Geometry: final body of the model. Coordinates: model frame, mm. A direction names the side the tool comes from. Round coordinates to 2 decimals unless told otherwise and drop trailing zeros. Order: outer loops, then holes, each group sorted by start corner. A loop starts at its lowest first (then second) coordinate and runs counter-clockwise, first axis right, second up. Notation, with made-up numbers: M 19.25,-16.75 L 53.25,-16.75 A10 cw 53.25,-7.75 Z; hole C 29,53 d8. An arc over 180 degrees is marked long. Return JSON: item names as keys, results as strings. Group by question number.
Q1. Mould query, pull axis X, two halves, no side actions, for faces 1 (the face through (42, 0, -136)), 2 (the face through (41, 3, -201.308)), 3 (the face through (87.336, 2, -136)), 4 (the face through (67, 3, -260.308)). Classes: released by +X, released by -X, zero draft, split by the parting line, or undercut.
Q2. Cut plane C-C on z = -68. Output: boundary loops of the cut face in (x, y), and give its area (3 significant figures).
Q3. Cut plane D-D on x = 32. Output: boundary loops of the cut face in (y, z), and give its area (3 significant figures).
Q4. Cut plane A-A on x = 20. Output: boundary loops of the cut face in (y, z), and give its area (3 significant figures).
Q5. Contact query for flat-ended pins moving along their axis: pin 1 (2.5 mm diameter, centred on x = 25.34, z = -194.31, fed in from -Y); pin 2 (5 mm diameter, centred on x = 25.34, z = -174.31, fed in from -Y). Output: stop coordinate, or through.
Q6. Ray query, probe 1 along Z at (x, y) = (46, 4.5); probe 2 along Z at (x, y) = (65, 2.4); probe 3 along X at (y, z) = (1, -227). Return the intervals inside material, ascending.
Q7. Cut plane B-B on z = -27. Output: boundary loops of the cut face in (x, y), and give its area (3 significant figures).
Q8. Access query for faces 5 (the face through (5.336, 3, -216)), 6 (the face through (42, 5, -136)). Directions: +Z, -Z, +X, -X, +Y, -Y. A direction counts if a zero-diameter tool reaches every point of the face in a straight line with its end or side. Return the directions, or none.
Autodesk Inventor part; units mm, degrees
ref_plane "YZ Plane" through (0, 0, 0) normal (1, 0, 0) x (0, 1, 0)
ref_plane "XZ Plane" through (0, 0, 0) normal (0, 1, 0) x (-1, 0, 0)
ref_plane "XY Plane" through (0, 0, 0) normal (0, 0, 1) x (1, 0, 0)
sketch "Sketch1" plane through (0, 0, 0) normal (0, 1, 0) x (-1, 0, 0)
  line L0 (4.6641, 6.6919) -> (-87.3359, 6.6919)
  line L1 (-87.3359, 6.6919) -> (-87.3359, -283.3081)
  line L2 (-87.3359, -283.3081) -> (4.6641, -283.3081)
  line L3 (4.6641, -283.3081) -> (4.6641, 6.6919)
  point P0 (0, 0)
  dimension "d0" = 290
  dimension "d1" = 92
extrude "Extrusion1" add sketch "Sketch1" along normal blind 5
sketch "Sketch2" plane through (0, 5, 0) normal (0, 1, 0) x (1, 0, 0)
  line L0 (-4.6641, 283.3081) -> (-4.6641, -6.6919)
  line L1 (87.3359, -6.6919) -> (87.3359, 283.3081)
  line L2 (9.3359, 45.3081) -> (73.3359, 45.3081)
  line L3 (77.3359, 49.3081) -> (77.3359, 71.3081)
  line L4 (73.3359, 75.3081) -> (9.3359, 75.3081)
  line L5 (5.3359, 71.3081) -> (5.3359, 49.3081)
  line L6 (-4.6641, -6.6919) -> (87.3359, -6.6919)
  arc A0 (5.3359, 49.3081) -> (9.3359, 45.3081) centre (9.3359, 49.3081) ccw
  arc A1 (9.3359, 75.3081) -> (5.3359, 71.3081) centre (9.3359, 71.3081) ccw
  arc A2 (77.3359, 71.3081) -> (73.3359, 75.3081) centre (73.3359, 71.3081) ccw
  arc A3 (73.3359, 45.3081) -> (77.3359, 49.3081) centre (73.3359, 49.3081) ccw
  line L7 (9.3359, 201.3081) -> (73.3359, 201.3081)
  line L8 (77.3359, 205.3081) -> (77.3359, 227.3081)
  line L9 (73.3359, 231.3081) -> (9.3359, 231.3081)
  line L10 (5.3359, 227.3081) -> (5.3359, 205.3081)
  arc A4 (5.3359, 205.3081) -> (9.3359, 201.3081) centre (9.3359, 205.3081) ccw
  arc A5 (9.3359, 231.3081) -> (5.3359, 227.3081) centre (9.3359, 227.3081) ccw
  arc A6 (77.3359, 227.3081) -> (73.3359, 231.3081) centre (73.3359, 227.3081) ccw
  arc A7 (73.3359, 201.3081) -> (77.3359, 205.3081) centre (73.3359, 205.3081) ccw
  line L11 (7.3359, 1.3081) -> (75.3359, 1.3081)
  line L12 (77.3359, 3.3081) -> (77.3359, 14.3081)
  line L13 (75.3359, 16.3081) -> (58.3359, 16.3081)
  line L14 (56.3359, 18.3081) -> (56.3359, 35.3081)
  line L15 (54.3359, 37.3081) -> (28.3359, 37.3081)
  line L16 (26.3359, 35.3081) -> (26.3359, 18.3081)
  line L17 (24.3359, 16.3081) -> (7.3359, 16.3081)
  line L18 (5.3359, 14.3081) -> (5.3359, 3.3081)
  arc A8 (5.3359, 3.3081) -> (7.3359, 1.3081) centre (7.3359, 3.3081) ccw
  arc A9 (7.3359, 16.3081) -> (5.3359, 14.3081) centre (7.3359, 14.3081) ccw
  arc A10 (24.3359, 16.3081) -> (26.3359, 18.3081) centre (24.3359, 18.3081) ccw
  arc A11 (28.3359, 37.3081) -> (26.3359, 35.3081) centre (28.3359, 35.3081) ccw
  arc A12 (56.3359, 35.3081) -> (54.3359, 37.3081) centre (54.3359, 35.3081) ccw
  arc A13 (56.3359, 18.3081) -> (58.3359, 16.3081) centre (58.3359, 18.3081) ccw
  arc A14 (77.3359, 14.3081) -> (75.3359, 16.3081) centre (75.3359, 14.3081) ccw
  arc A15 (75.3359, 1.3081) -> (77.3359, 3.3081) centre (75.3359, 3.3081) ccw
  line L19 (87.3359, 283.3081) -> (-4.6641, 283.3081)
  line L20 (5.3359, 273.3081) -> (5.3359, 262.3081)
  line L21 (7.3359, 260.3081) -> (24.3359, 260.3081)
  line L22 (26.3359, 258.3081) -> (26.3359, 241.3081)
  line L23 (28.3359, 239.3081) -> (54.3359, 239.3081)
  line L24 (56.3359, 241.3081) -> (56.3359, 258.3081)
  line L25 (58.3359, 260.3081) -> (75.3359, 260.3081)
  line L26 (77.3359, 262.3081) -> (77.3359, 273.3081)
  line L27 (75.3359, 275.3081) -> (7.3359, 275.3081)
  arc A16 (26.3359, 258.3081) -> (24.3359, 260.3081) centre (24.3359, 258.3081) ccw
  arc A17 (5.3359, 262.3081) -> (7.3359, 260.3081) centre (7.3359, 262.3081) ccw
  arc A18 (7.3359, 275.3081) -> (5.3359, 273.3081) centre (7.3359, 273.3081) ccw
  arc A19 (77.3359, 273.3081) -> (75.3359, 275.3081) centre (75.3359, 273.3081) ccw
  arc A20 (75.3359, 260.3081) -> (77.3359, 262.3081) centre (75.3359, 262.3081) ccw
  arc A21 (58.3359, 260.3081) -> (56.3359, 258.3081) centre (58.3359, 258.3081) ccw
  arc A22 (54.3359, 239.3081) -> (56.3359, 241.3081) centre (54.3359, 241.3081) ccw
  arc A23 (26.3359, 241.3081) -> (28.3359, 239.3081) centre (28.3359, 241.3081) ccw
  point P0 (5.3359, 45.3081)
  point P1 (77.3359, 75.3081)
  point P2 (5.3359, 75.3081)
  point P3 (5.3359, 201.3081)
  point P4 (77.3359, 201.3081)
  point P5 (5.3359, 231.3081)
  point P6 (5.3359, 1.3081)
  point P7 (77.3359, 1.3081)
  point P8 (77.3359, 16.3081)
  point P9 (56.3359, 16.3081)
  point P10 (26.3359, 16.3081)
  point P11 (5.3359, 16.3081)
  point P12 (5.3359, 275.3081)
  point P13 (5.3359, 260.3081)
  point P14 (26.3359, 260.3081)
  point P15 (56.3359, 260.3081)
  point P16 (77.3359, 260.3081)
  point P17 (77.3359, 275.3081)
  dimension "d12" = 30
  dimension "d13" = 72
  dimension "d14" = 10
  dimension "d16" = 4
  dimension "d17" = 30
  dimension "d18" = 10
  dimension "d19" = 72
  dimension "d21" = 4
  dimension "d41" = 10
  dimension "d42" = 72
  dimension "d43" = 15
  dimension "d44" = 21
  dimension "d45" = 21
  dimension "d46" = 36
  dimension "d47" = 15
  dimension "d48" = 8
  dimension "d49" = 2
  dimension "d58" = 10
  dimension "d59" = 8
  dimension "d60" = 72
  dimension "d61" = 15
  dimension "d62" = 36
  dimension "d63" = 21
  dimension "d64" = 21
  dimension "d65" = 2
  dimension "d66" = 2
  dimension "d170" = 8
  dimension "d171" = 8
extrude "Extrusion2" cut sketch "Sketch2" against normal up to next contours A0 L5 A1 L4 A2 L3 A3 L2 | A4 L10 A5 L9 A6 L8 A7 L7 | A8 L18 A9 L17 A10 L16 A11 L15 A12 L14 A13 L13 A14 L12 A15 L11 | A18 L27 A19 L26 A20 L25 A21 L24 A22 L23 A23 L22 A16 L21 A17 L20
sketch "Sketch3" plane through (0, 5, 0) normal (0, 1, 0) x (1, 0, 0)
  circle A0 centre (0.3359, -1.6919) radius 1.5
  circle A1 centre (82.3359, -1.6919) radius 1.5
  circle A2 centre (0.3359, 83.3081) radius 1.5
  circle A3 centre (0.3359, 138.3081) radius 1.5
  circle A4 centre (0.3359, 193.3081) radius 1.5
  circle A5 centre (0.3359, 278.3081) radius 1.5
  circle A6 centre (82.3359, 83.3081) radius 1.5
  circle A7 centre (82.3359, 138.3081) radius 1.5
  circle A8 centre (82.3359, 193.3081) radius 1.5
  circle A9 centre (82.3359, 278.3081) radius 1.5
  line L0 (-4.6641, -6.6919) -> (87.3359, -6.6919)
  line L1 (-4.6641, 283.3081) -> (-4.6641, -6.6919)
  line L2 (87.3359, -6.6919) -> (87.3359, 283.3081)
  line L3 (87.3359, 283.3081) -> (-4.6641, 283.3081)
  circle A10 centre (82.3359, 21.3081) radius 1
  circle A11 centre (67.3359, 21.3081) radius 1
  circle A12 centre (82.3359, 255.3081) radius 1
  circle A13 centre (67.3359, 255.3081) radius 1
  circle A14 centre (25.3359, 82.3081) radius 1.5
  circle A15 centre (25.3359, 102.3081) radius 1.5
  circle A16 centre (57.3359, 82.3081) radius 1.5
  circle A17 centre (57.3359, 102.3081) radius 1.5
  circle A18 centre (25.3359, 194.3081) radius 1.5
  circle A19 centre (25.3359, 174.3081) radius 1.5
  circle A20 centre (57.3359, 194.3081) radius 1.5
  circle A21 centre (57.3359, 174.3081) radius 1.5
  line L4 (9.3359, 75.3081) -> (73.3359, 75.3081)
  line L5 (73.3359, 201.3081) -> (9.3359, 201.3081)
  circle A22 centre (57.3359, 122.3081) radius 1.5
  circle A23 centre (25.3359, 122.3081) radius 1.5
  circle A24 centre (25.3359, 154.3081) radius 1.5
  circle A25 centre (57.3359, 154.3081) radius 1.5
  line L6 (75.3359, 260.3081) -> (58.3359, 260.3081)
  line L7 (58.3359, 16.3081) -> (75.3359, 16.3081)
  circle A26 centre (8.8359, 18.8081) radius 1
  circle A27 centre (13.8359, 18.8081) radius 1
  line L8 (26.3359, 18.3081) -> (26.3359, 35.3081)
  line L9 (7.3359, 16.3081) -> (24.3359, 16.3081)
  circle A28 centre (13.8359, 257.8081) radius 1
  circle A29 centre (8.8359, 257.8081) radius 1
  line L10 (26.3359, 241.3081) -> (26.3359, 258.3081)
  line L11 (24.3359, 260.3081) -> (7.3359, 260.3081)
  point P0 (0, 0)
  dimension "d70" = 3
  dimension "d71" = 5
  dimension "d72" = 5
  dimension "d73" = 3
  dimension "d74" = 5
  dimension "d75" = 5
  dimension "d77" = 3
  dimension "d78" = 3
  dimension "d79" = 3
  dimension "d81" = 3
  dimension "d82" = 3
  dimension "d84" = 3
  dimension "d85" = 3
  dimension "d86" = 3
  dimension "d89" = 5
  dimension "d90" = 5
  dimension "d91" = 5
  dimension "d93" = 5
  dimension "d95" = 5
  dimension "d96" = 5
  dimension "d97" = 5
  dimension "d99" = 5
  dimension "d100" = 5
  dimension "d101" = 5
  dimension "d106" = 145
  dimension "d107" = 145
  dimension "d108" = 90
  dimension "d109" = 90
  dimension "d110" = 90
  dimension "d111" = 90
  dimension "d112" = 2
  dimension "d113" = 2
  dimension "d114" = 2
  dimension "d115" = 2
  dimension "d116" = 5
  dimension "d119" = 20
  dimension "d120" = 5
  dimension "d121" = 20
  dimension "d124" = 3
  dimension "d125" = 3
  dimension "d127" = 3
  dimension "d128" = 3
  dimension "d131" = 3
  dimension "d132" = 3
  dimension "d133" = 3
  dimension "d134" = 3
  dimension "d136" = 30
  dimension "d137" = 30
  dimension "d139" = 30
  dimension "d140" = 30
  dimension "d143" = 30
  dimension "d144" = 30
  dimension "d145" = 30
  dimension "d146" = 30
  dimension "d148" = 7
  dimension "d149" = 7
  dimension "d150" = 7
  dimension "d151" = 7
  dimension "d152" = 20
  dimension "d153" = 3
  dimension "d154" = 30
  dimension "d155" = 20
  dimension "d156" = 20
  dimension "d157" = 3
extrude "Extrusion3" cut sketch "Sketch3" against normal blind 5 contours A0 | A1 | A2 | A3 | A4 | A5 | A6 | A7 | A8 | A9 | A10 | A11 | A12 | A13 | A14 | A15 | A16 | A17 | A18 | A19 | A20 | A21 | A22 | A23 | A24 | A25 | A26 | A27 | A28 | A29
properties part number "base_roulante"
Result sheet:
{
 "1": {"face 1": "zero draft", "face 2": "undercut", "face 3": "released by +X", "face 4": "undercut"},
 "2": {"outline": "M -4.66,0 L 5.34,0 L 5.34,5 L -4.66,5 Z; M 77.34,0 L 87.34,0 L 87.34,5 L 77.34,5 Z", "area": "100 mm²"},
 "3": {"outline": "M 0,-283.31 L 5,-283.31 L 5,-275.31 L 0,-275.31 Z; M 0,-239.31 L 5,-239.31 L 5,-231.31 L 0,-231.31 Z; M 0,-201.31 L 5,-201.31 L 5,-75.31 L 0,-75.31 Z; M 0,-45.31 L 5,-45.31 L 5,-37.31 L 0,-37.31 Z; M 0,-1.31 L 5,-1.31 L 5,6.69 L 0,6.69 Z", "area": "790 mm²"},
 "4": {"outline": "M 0,-283.31 L 5,-283.31 L 5,-275.31 L 0,-275.31 Z; M 0,-260.31 L 5,-260.31 L 5,-231.31 L 0,-231.31 Z; M 0,-201.31 L 5,-201.31 L 5,-75.31 L 0,-75.31 Z; M 0,-45.31 L 5,-45.31 L 5,-16.31 L 0,-16.31 Z; M 0,-1.31 L 5,-1.31 L 5,6.69 L 0,6.69 Z", "area": "1,000 mm²"},
 "5": {"pin 1": "passes through", "pin 2": "stops at y = 0"},
 "6": {"probe 1": "z = -283.31 to -275.31, -239.31 to -231.31, -201.31 to -75.31, -45.31 to -37.31, -1.31 to 6.69", "probe 2": "z = -283.31 to -275.31, -260.31 to -231.31, -201.31 to -75.31, -45.31 to -16.31, -1.31 to 6.69", "probe 3": "x = -4.66 to 5.34, 77.34 to 87.34"},
 "7": {"outline": "M -4.66,0 L 26.34,0 L 26.34,5 L -4.66,5 Z; M 56.34,0 L 87.34,0 L 87.34,5 L 56.34,5 Z", "area": "310 mm²"},
 "8": {"face 5": "+Y, -Y", "face 6": "+Z, -Z, +X, -X, +Y"}
}
